from build123d import *

# Parameters (mm, degrees)
SKETCH1_R           = 1.5
BOSS_EXTRUDE1_DEPTH = 10
CUT_EXTRUDE2_DEPTH  = 3
SKETCH3_R           = 7.5
SKETCH3_R_2         = 6.5
BOSS_EXTRUDE2_DEPTH = 90
CHAMFER1_SIZE       = 3


with BuildPart() as part:
    # Sketch1 → Boss-Extrude1 (new body)
    with BuildSketch(Plane.XY):
        with BuildLine():
            Line((-13.009713205, 28.5), (13.009713205, 28.5))
            ThreePointArc((13.009713205, 28.5), (14.59383519, 27.84383519), (15.25, 26.259713205))
            Line((15.25, 26.259713205), (15.25, 2.240286795))
            ThreePointArc((15.25, 2.240286795), (14.59383519, 0.65616481), (13.009713205, 0))
            Line((13.009713205, 0), (-13.009713205, 0))
            ThreePointArc((-13.009713205, 0), (-14.59383519, 0.65616481), (-15.25, 2.240286795))
            Line((-15.25, 2.240286795), (-15.25, 26.259713205))
            ThreePointArc((-15.25, 26.259713205), (-14.59383519, 27.84383519), (-13.009713205, 28.5))
        make_face()
        with Locations((-10.5, 20.25)):
            Circle(SKETCH1_R, mode=Mode.SUBTRACT)
        with Locations((10.5, 20.25)):
            Circle(SKETCH1_R, mode=Mode.SUBTRACT)
        with Locations((10.5, 8.25)):
            Circle(SKETCH1_R, mode=Mode.SUBTRACT)
        with Locations((-10.5, 8.25)):
            Circle(SKETCH1_R, mode=Mode.SUBTRACT)
    extrude(amount=BOSS_EXTRUDE1_DEPTH)

    # Sketch2 → Cut-Extrude2 (cut)
    with BuildSketch(Plane.XY.offset(10)):
        Polygon((-10.5, 23.425426481), (-13.25, 21.83771324), (-13.25, 18.66228676), (-10.5, 17.074573519), (-7.75, 18.66228676), (-7.75, 21.83771324), align=None)
        Polygon((-10.5, 11.425426481), (-13.25, 9.83771324), (-13.25, 6.66228676), (-10.5, 5.074573519), (-7.75, 6.66228676), (-7.75, 9.83771324), align=None)
        Polygon((10.5, 23.425426481), (7.75, 21.83771324), (7.75, 18.66228676), (10.5, 17.074573519), (13.25, 18.66228676), (13.25, 21.83771324), align=None)
        Polygon((10.5, 11.425426481), (7.75, 9.83771324), (7.75, 6.66228676), (10.5, 5.074573519), (13.25, 6.66228676), (13.25, 9.83771324), align=None)
    extrude(amount=-CUT_EXTRUDE2_DEPTH, mode=Mode.SUBTRACT)

    # Sketch3 → Boss-Extrude2 (add)
    with BuildSketch(Plane.XY.offset(10)):
        with Locations(Location((0, 14.25, 0), (0, 0, 180))):
            Circle(SKETCH3_R)
        with Locations(Location((0, 14.25, 0), (0, 0, 180))):
            Circle(SKETCH3_R_2, mode=Mode.SUBTRACT)
    extrude(amount=BOSS_EXTRUDE2_DEPTH)

    # Chamfer1
    # the kernel refuses this chamfer: 3 mm, written as the material it adds along each edge
    with BuildSketch(Plane(origin=(0, 14.25, 10), x_dir=(-1, 0, 0), z_dir=(0, 1, 0))) as chamfer1_piece_1_section:
        Polygon((7.5 + CHAMFER1_SIZE, 0), (7.5, CHAMFER1_SIZE), (7.5, 0), align=None)
    chamfer1_piece_1 = revolve(axis=Axis((0, 14.25, 10), (0, 0, 1)), mode=Mode.PRIVATE)
    chamfer1_piece_1 = split(chamfer1_piece_1, bisect_by=Plane(origin=(7.75, 14.25, 10.835375001), z_dir=(-1, 0, 0)), keep=Keep.TOP, mode=Mode.PRIVATE)
    chamfer1_piece_1 = split(chamfer1_piece_1, bisect_by=Plane(origin=(-10.27932295, 11.298018527, 10.835375001), z_dir=(0.4999999999999999, 0.8660254037844388, 0)), keep=Keep.TOP, mode=Mode.PRIVATE)
    chamfer1_piece_1 = split(chamfer1_piece_1, bisect_by=Plane(origin=(-10.27932295, 17.201981474, 10.835375001), z_dir=(0.5000000000000004, -0.8660254037844384, 0)), keep=Keep.TOP, mode=Mode.PRIVATE)
    add(chamfer1_piece_1)
    with BuildSketch(Plane(origin=(0, 14.25, 10), x_dir=(-1, 0, 0), z_dir=(0, 1, 0))) as chamfer1_piece_2_section:
        Polygon((7.5 + CHAMFER1_SIZE, 0), (7.5, CHAMFER1_SIZE), (7.5, 0), align=None)
    chamfer1_piece_2 = revolve(axis=Axis((0, 14.25, 10), (0, 0, 1)), mode=Mode.PRIVATE)
    chamfer1_piece_2 = split(chamfer1_piece_2, bisect_by=Plane(origin=(7.75, 21.633797899, 10.850650839), z_dir=(-1, 0, 0)), keep=Keep.TOP, mode=Mode.PRIVATE)
    chamfer1_piece_2 = split(chamfer1_piece_2, bisect_by=Plane(origin=(-7.75, 21.633797899, 10.850650839), z_dir=(1, 0, 0)), keep=Keep.TOP, mode=Mode.PRIVATE)
    add(chamfer1_piece_2)
    with BuildSketch(Plane(origin=(0, 14.25, 10), x_dir=(-1, 0, 0), z_dir=(0, 1, 0))) as chamfer1_piece_3_section:
        Polygon((7.5 + CHAMFER1_SIZE, 0), (7.5, CHAMFER1_SIZE), (7.5, 0), align=None)
    chamfer1_piece_3 = revolve(axis=Axis((0, 14.25, 10), (0, 0, 1)), mode=Mode.PRIVATE)
    chamfer1_piece_3 = split(chamfer1_piece_3, bisect_by=Plane(origin=(10.279322953, 11.298018528, 10.835374999), z_dir=(-0.5000000000000011, 0.866025403784438, 0)), keep=Keep.TOP, mode=Mode.PRIVATE)
    chamfer1_piece_3 = split(chamfer1_piece_3, bisect_by=Plane(origin=(-7.75, 14.25, 10.835374999), z_dir=(1, 0, 0)), keep=Keep.TOP, mode=Mode.PRIVATE)
    chamfer1_piece_3 = split(chamfer1_piece_3, bisect_by=Plane(origin=(10.279322953, 17.201981472, 10.835374999), z_dir=(-0.49999999999999445, -0.8660254037844419, 0)), keep=Keep.TOP, mode=Mode.PRIVATE)
    add(chamfer1_piece_3)


solid = part.part
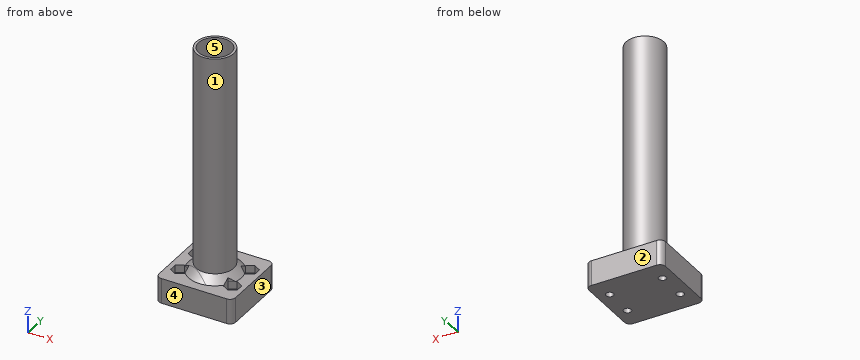
Design review of the part built by this model. Coordinates are the model's own, in mm. Face numbers are marked on the shaded views. A direction names the side the tool comes from. Give positions to 0.01 mm unless a question says otherwise; leave off trailing zeros. Order: outer loops, then holes, each group sorted by start corner. A loop starts at its lowest first (then second) coordinate and runs counter-clockwise, first axis right, second up. Notation, with made-up numbers: (-16, 59.25) - (31, 59.25) arc R29 cw to (31, 79.25) - close; hole circle Ø10 at (21, 22). An arc over 180 degrees is marked (long way). Use CSV: the item, a comma, the result in double quotes. Start each with the question number.
Q1. Take a section at B-B (z = 17). State the section outline as (x, y) points, and give its area (3 significant figures).
Q2. Take a section at A-A (y = 14.25). State the section outline as (x, z) points, and give its area (3 significant figures).
Q3. Draft analysis for pull direction Y (two halves, no side actions). For the marked faces 3, 4 and 5, state which applies: pulls with the +Y half, pulls with the -Y half, needs draft (parallel to the pull), parting line crosses it, or undercut.
Q4. For P1, Ø3, axis at x = -10.5, y = 19.5, coming from the +Z side; P2, Ø5, axis at y = 19.5, z = 81.5, coming from the -X side; P3, Ø12, axis at x = -9, z = 26.5, coming from the -Y side; P4, Ø6, axis at x = -3.5, y = 17, coming from the +Z side, all flat-tipped, find the tip position at first contact; note any pin that passes through.
Q5. For line 1 (X direction, y = 20.25, z = 3); line 2 (X direction, y = 7.75, z = 8); line 3 (Y direction, x = 0, z = 83.5), list the stretches that pass through material, from the lowest coordinate up.
Q6. Machinability: for the marked faces 1 and 2, which of the approach directions +Z, -Z, +X, -X, +Y, -Y give a long, thin tool a straight path to every point of the face, cutting with its end or side? Answer none if there is none.
Calculated:
1,outline,"circle Ø15 at (0, 14.25); hole circle Ø13 at (0, 14.25)"
1,area,"44.0 mm²"
2,outline,"(-15.25, 0) - (15.25, 0) - (15.25, 10) - (10.5, 10) - (7.5, 13) - (7.5, 100) - (6.5, 100) - (6.5, 10) - (-6.5, 10) - (-6.5, 100) - (-7.5, 100) - (-7.5, 13) - (-10.5, 10) - (-15.25, 10) - close"
2,area,"494 mm²"
3,face 3,"needs draft"
3,face 4,"pulls with the -Y half"
3,face 5,"undercut"
4,P1,"stops at z = 7"
4,P2,"stops at x = -6.98"
4,P3,"stops at y = 7.38"
4,P4,"stops at z = 100"
5,line 1,"x = -15.25 to -12, -9 to 9, 12 to 15.25"
5,line 2,"x = -15.25 to -13.25, -7.75 to 7.75, 13.25 to 15.25"
5,line 3,"y = 6.75 to 7.75, 20.75 to 21.75"
6,face 1,"+Z"
6,face 2,"+Z, -Z, +X, -X, +Y"
